Model file for the job. Use its own axes, mm. Face numbers are marked on the shaded views. A direction names the side the tool comes from. Round coordinates to 2 decimals unless told otherwise and drop trailing zeros. Write each loop counter-clockwise with the first axis right and the second up, starting at its lowest first coordinate (ties: lowest second). Pieces come first, ordered by that corner, then holes.
```python
from build123d import *

# Parameters (mm, degrees)
BOSS_EXTRU_1_DEPTH         = 10
ESQUISSE2_R                = 1.5
ENL_V_MAT_EXTRU_1_DEPTH    = 33.5
R_P_TITION_LIN_AIRE1_COUNT = 2
R_P_TITION_LIN_AIRE1_PITCH = 10
ESQUISSE3_R                = 1.5
ENL_V_MAT_EXTRU_2_DEPTH    = 33.5
R_P_TITION_LIN_AIRE2_COUNT = 2
R_P_TITION_LIN_AIRE2_PITCH = 10


with BuildPart() as part:
    # Esquisse1 → Boss.-Extru.1 (new body)
    with BuildSketch(Plane.XY):
        Polygon((0, 0), (32.5, 0), (32.5, 1), (1, 1), (1, 32.5), (0, 32.5), align=None)
    extrude(amount=BOSS_EXTRU_1_DEPTH)

    # Esquisse2 → Enlèv. mat.-Extru.1 (cut, through all)
    with BuildSketch(Plane.ZY):
        with Locations((5, 27.5)):
            Circle(ESQUISSE2_R)
    enl_v_mat_extru_1 = extrude(amount=-ENL_V_MAT_EXTRU_1_DEPTH, mode=Mode.SUBTRACT)

    # Répétition linéaire1: Enlèv. mat.-Extru.1 ×2
    with Locations(*[(0, -i * R_P_TITION_LIN_AIRE1_PITCH, 0) for i in range(1, R_P_TITION_LIN_AIRE1_COUNT)]):
        add(enl_v_mat_extru_1, mode=Mode.SUBTRACT)

    # Esquisse3 → Enlèv. mat.-Extru.2 (cut, through all)
    with BuildSketch(Plane.XZ):
        with Locations((27.5, 5)):
            Circle(ESQUISSE3_R)
    enl_v_mat_extru_2 = extrude(amount=-ENL_V_MAT_EXTRU_2_DEPTH, mode=Mode.SUBTRACT)

    # Répétition linéaire2: Enlèv. mat.-Extru.2 ×2
    with Locations(*[(-i * R_P_TITION_LIN_AIRE2_PITCH, 0, 0) for i in range(1, R_P_TITION_LIN_AIRE2_COUNT)]):
        add(enl_v_mat_extru_2, mode=Mode.SUBTRACT)


solid = part.part
```
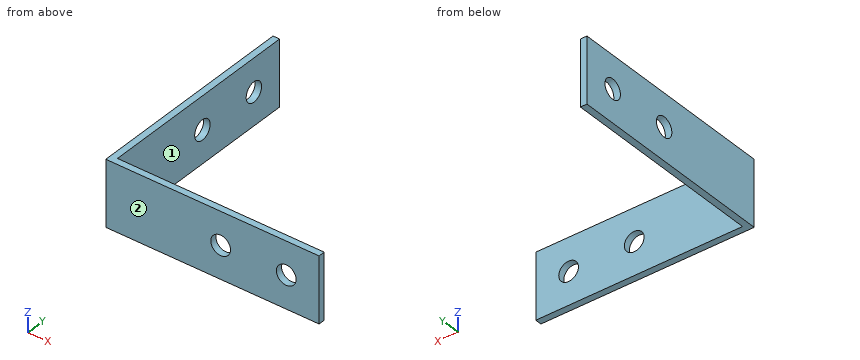
1) Which spindle directions (+Z, -Z, +X, -X, +Y, -Y) get a long thin tool onto all of the face, cutting with end or side? Do the marked faces 1 and 2. Say none if no direction does.
2) Cut at C-C on z = 5. List the corners of the cut face in (x, y).
3) Cut at A-A on x = 27.5. List the corners of the cut face in (y, z).
4) Cut at D-D on z = 1.25. List the corners of the cut face in (x, y).
5) Wall check: probe 1 along Y at (x, z) = (0.55, 5); probe 2 along Z at (x, y) = (17.5, 0.4); probe 3 along X at (y, z) = (20, 4). Give the ranges that are in metal, low to high.
6) Flat gauge pins, fed straight in: pin 1 Ø6 at (x, z) = (25.5, 7) entering from -Y; pin 2 Ø5 at (x, z) = (11.5, 3.5) entering from +Y; pin 3 Ø4 at (y, z) = (27.5, 5) entering from +X. Where does each tip first touch, or does it go through?
Result sheet:
1. face 1: +Z, -Z, +X, +Y
1. face 2: +Z, -Z, +X, -X, -Y
2. outline: (0, 0) - (16, 0) - (16, 1) - (1, 1) - (1, 16) - (0, 16) - close; (0, 19) - (1, 19) - (1, 26) - (0, 26) - close; (0, 29) - (1, 29) - (1, 32.5) - (0, 32.5) - close; (19, 0) - (26, 0) - (26, 1) - (19, 1) - close; (29, 0) - (32.5, 0) - (32.5, 1) - (29, 1) - close
3. outline: (0, 0) - (1, 0) - (1, 3.5) - (0, 3.5) - close; (0, 6.5) - (1, 6.5) - (1, 10) - (0, 10) - close
4. outline: (0, 0) - (32.5, 0) - (32.5, 1) - (1, 1) - (1, 32.5) - (0, 32.5) - close
5. probe 1: y = 0 to 16, 19 to 26, 29 to 32.5
5. probe 2: z = 0 to 3.5, 6.5 to 10
5. probe 3: x = 0 to 1
6. pin 1: stops at y = 0
6. pin 2: stops at y = 1
6. pin 3: stops at x = 1
